Geometry: see drawing. Coordinates: mm, zero at the bounding-box minimum. Coordinates: 2 decimals unless noted, no trailing zeros. Order: outer loops, then holes, each group sorted by start corner. A loop starts at its lowest first (then second) coordinate and runs counter-clockwise, first axis right, second up. Notation, with made-up numbers: (17.25, -37) -> (69.25, -37) arc R31 ccw to (69.25, -13) -> close; hole circle Ø11 at (58.25, 48). An arc over 180 degrees is marked (long way). One line per item, written item: value. Start each with the question number.
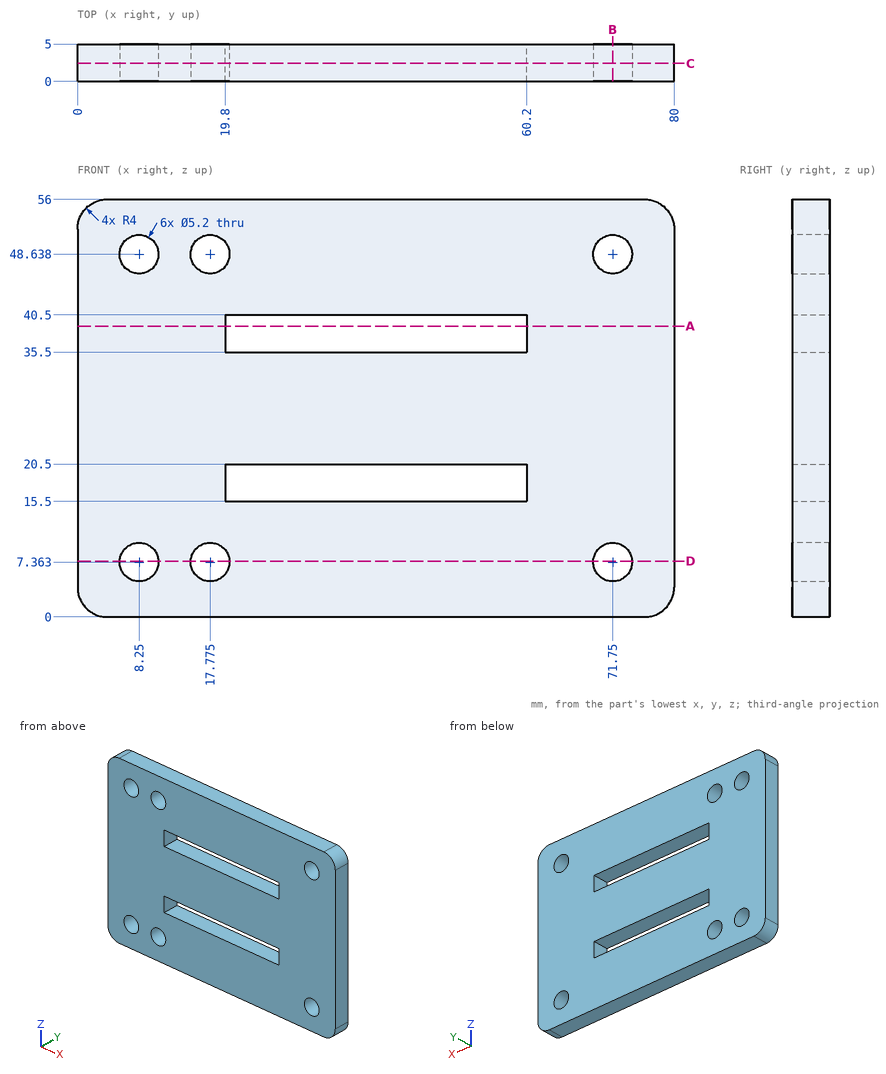
1) Section query B-B, the plane x = 71.75. Return the cut outline in (y, z), plus the area to 3 significant figures.
2) Section query D-D, the plane z = 7.5. Return the cut outline in (x, y), plus the area to 3 significant figures.
3) Section query A-A, the plane z = 39. Return the cut outline in (x, y).
4) Section query C-C, the plane y = 2.4. State how many separate pieces and enclosed holes the cut face has.
5) Ray query, line 1 along Z through (x, y) = (8.25, 3.1); line 2 along Z through (x, y) = (39, 2.4); line 3 along X through (y, z) = (0.4, 16). Return the intervals inside material, ascending. Write a range as from..to.
Entries:
1. outline: (0, 0) -> (5, 0) -> (5, 4.76) -> (0, 4.76) -> close; (0, 9.96) -> (5, 9.96) -> (5, 46.04) -> (0, 46.04) -> close; (0, 51.24) -> (5, 51.24) -> (5, 56) -> (0, 56) -> close
1. area: 228 mm2
2. outline: (0, 0) -> (5.65, 0) -> (5.65, 5) -> (0, 5) -> close; (10.85, 0) -> (15.18, 0) -> (15.18, 5) -> (10.85, 5) -> close; (20.37, 0) -> (69.15, 0) -> (69.15, 5) -> (20.37, 5) -> close; (74.35, 0) -> (80, 0) -> (80, 5) -> (74.35, 5) -> close
2. area: 322 mm2
3. outline: (0, 0) -> (19.8, 0) -> (19.8, 5) -> (0, 5) -> close; (60.2, 0) -> (80, 0) -> (80, 5) -> (60.2, 5) -> close
4. separate pieces: 1
4. enclosed holes: 8
5. line 1: z = 0..4.76, 9.96..46.04, 51.24..56
5. line 2: z = 0..15.5, 20.5..35.5, 40.5..56
5. line 3: x = 0..19.8, 60.2..80
